The model under review builds one solid part; all positions refer to its coordinate system, in mm. A direction names the side the tool comes from. Round coordinates to 2 decimals unless told otherwise and drop trailing zeros. Order: outer loops, then holes, each group sorted by start corner. A loop starts at its lowest first (then second) coordinate and runs counter-clockwise, first axis right, second up.
1) Consider section D-D (z = -69.5). Give the boundary of the cut face in (x, y), then the cut area to 3 significant figures.
2) Clearance check with flat-ended pins moving along their axes: P1, Ø6, axis at x = -43.5, z = 28.5, coming from the -Y side; P2, Ø2, axis at x = -41.5, y = 4.5, coming from the -Z side; P3, Ø3, axis at y = 2, z = 62.5, coming from the +X side; P4, Ø1, axis at y = 1, z = 46.5, coming from the +X side. State where each tip first meets the part, or that it passes through.
3) Mouldability with a two-part tool opening along X and no side actions: class faces 1 (the face through (64.235, 3.131, -35.389)), 2 (the face through (23.54, 3.219, -86.914)), 3 (the face through (-0.186, 3.219, -133.946)) as pulls with the +X half, pulls with the -X half, needs draft (parallel to the pull), parting line crosses it, or undercut.
4) Consider section B-B (y = 3). Give the number of separate pieces and of enclosed holes in the cut face, then the cut area to 3 significant figures.
5) To check wall thickness, follow L1, parallel to X at y = 2.5, z = -85.5; L2, parallel to X at y = 1, z = 15; L3, parallel to X at y = 0.5, z = 16.5. State the ranges of each line that lie inside material, in increasing order.
6) Consider section A-A (z = 32). Give the boundary of the cut face in (x, y).
7) Machinability: for faces 4 (the face through (86.62, 3.22, 16.08)), 5 (the face through (-116.1, 3.2, 66.8)), which of the approach directions +Z, -Z, +X, -X, +Y, -Y give a long, thin tool a straight path to every point of the face, cutting with its end or side? Answer none if there is none.
8) Consider section C-C (x = -70). Give the boundary of the cut face in (y, z).
from build123d import *

# Parameters (mm, degrees)
BOSS_EXTRUDE1_DEPTH = 6.35
SKETCH2_W           = 36.5
SKETCH2_H           = 63
SKETCH2_R           = 1.4224
CUT_EXTRUDE2_DEPTH  = 195.099602868
FILLET1_R           = 12.7
SKETCH3_W           = 12.7
SKETCH3_H           = 6.35
CUT_EXTRUDE3_DEPTH  = 179.426731159


with BuildPart() as part:
    # Sketch1 → Boss-Extrude1 (new body)
    with BuildSketch(Plane(origin=(0, 0, 0), x_dir=(1, 0, 0), z_dir=(0, 1, 0))):
        Polygon((0, 146.646968374), (-127, -73.323484187), (127, -73.323484187), align=None)
    extrude(amount=BOSS_EXTRUDE1_DEPTH)

    # Sketch2 → Cut-Extrude2 (cut, through all)
    with BuildSketch(Plane(origin=(0, 6.35, 0), x_dir=(1, 0, 0), z_dir=(0, 1, 0))):
        with Locations((-18.25, -24.043484187)):
            Rectangle(SKETCH2_W, SKETCH2_H)
        with Locations((18.25, -24.043484187)):
            Rectangle(SKETCH2_W, SKETCH2_H)
        with Locations(Location((0, 118.312139176, 0), (0, 0, 270))):
            Circle(SKETCH2_R)
        with Locations(Location((-102.461318102, -59.156069588, 0), (0, 0, 270))):
            Circle(SKETCH2_R)
        with Locations(Location((102.461318102, -59.156069588, 0), (0, 0, 270))):
            Circle(SKETCH2_R)
    extrude(amount=-CUT_EXTRUDE2_DEPTH, mode=Mode.SUBTRACT)

    # Fillet1
    fillet1_edges = [part.edges().sort_by_distance(p)[0] for p in [
        (127, 3.175, 73.323484187),
        (-127, 3.175, 73.323484187),
        (0, 3.175, -146.646968374),
    ]]
    fillet(fillet1_edges, radius=FILLET1_R)

    # Sketch3 → Cut-Extrude3 (cut, through all)
    with BuildSketch(Plane(origin=(0, 6.35, 0), x_dir=(1, 0, 0), z_dir=(0, 1, 0))):
        Polygon((-26.250738686, 88.479355234), (-32.600738686, 77.480832606), (-27.101477372, 74.305832606), (-20.751477372, 85.304355234), align=None)
        Polygon((-77.901477372, -13.682348419), (-83.400738686, -10.507348419), (-89.750738686, -21.505871047), (-84.251477372, -24.680871047), align=None)
        with Locations((-57.15, -63.798484187)):
            Rectangle(SKETCH3_W, SKETCH3_H)
        with Locations((57.15, -63.798484187)):
            Rectangle(SKETCH3_W, SKETCH3_H)
        Polygon((89.750738686, -21.505871047), (83.400738686, -10.507348419), (77.901477372, -13.682348419), (84.251477372, -24.680871047), align=None)
        Polygon((27.101477372, 74.305832606), (32.600738686, 77.480832606), (26.250738686, 88.479355234), (20.751477372, 85.304355234), align=None)
    extrude(amount=-CUT_EXTRUDE3_DEPTH, mode=Mode.SUBTRACT)


solid = part.part
Answer below:
1. outline: (-44.54, 0) - (44.54, 0) - (44.54, 6.35) - (-44.54, 6.35) - close
1. area: 566 mm2
2. P1: stops at y = 0
2. P2: stops at z = -76.5
2. P3: stops at x = 117.7
2. P4: stops at x = 111.8
3. face 1: pulls with the +X half
3. face 2: undercut
3. face 3: parting line crosses it
4. separate pieces: 1
4. enclosed holes: 10
4. area: 22,500 mm2
5. L1: x = -35.3 to -27.97, -21.09 to 21.09, 27.97 to 35.3
5. L2: x = -93.33 to -85.99, -78.66 to -36.5, 36.5 to 78.66, 85.99 to 93.33
5. L3: x = -94.19 to -86.86, -79.53 to -36.5, 36.5 to 79.53, 86.86 to 94.19
6. outline: (-103.14, 0) - (-36.5, 0) - (-36.5, 6.35) - (-103.14, 6.35) - close; (36.5, 0) - (103.14, 0) - (103.14, 6.35) - (36.5, 6.35) - close
7. face 4: +Y, -Y
7. face 5: -X, +Y, -Y
8. outline: (0, -25.4) - (6.35, -25.4) - (6.35, 73.32) - (0, 73.32) - close
